Could you check a few things on this model? Use its own coordinates, in mm. A direction names the side the tool comes from. Round coordinates to 2 decimals unless told otherwise and drop trailing zeros. Loops run counter-clockwise (first coordinate to the right, second up) from the corner with the lowest first, then second, coordinate; pieces in that order, holes last. Notation, with made-up numbers: M 36.25,-33.75 L 73.25,-33.75 A24 cw 73.25,2.25 Z; hole C -27,-8.75 d10. An arc over 180 degrees is marked long. Return JSON: item names as keys, results as strings. Group by question number.
```python
from build123d import *

# Parameters (mm, degrees)
F1_DEPTH = 6.35
F2_R     = 2.38125
F3_DEPTH = 6.35


with BuildPart() as f1:
    # F0 (on Top) → F1 (new body)
    with BuildSketch(Plane.XY):
        with BuildLine():
            Line((-9.525, 10.649274), (-6.35, 7.099516))
            ThreePointArc((-6.35, 7.099516), (9.525, 0), (-6.35, -7.099516))
            Line((-6.35, -7.099516), (-9.525, -10.649274))
            ThreePointArc((-9.525, -10.649274), (14.2875, 0), (-9.525, 10.649274))
        make_face()
    extrude(amount=F1_DEPTH)

    # F2 (on Top) → F3 (join, through all)
    with BuildSketch(Plane.XY):
        with BuildLine():
            Line((39.330256, 3.175), (13.930256, 3.175))
            ThreePointArc((13.930256, 3.175), (14.2875, 0), (13.930256, -3.175))
            Line((13.930256, -3.175), (39.330256, -3.175))
            ThreePointArc((39.330256, -3.175), (42.505256, 0), (39.330256, 3.175))
        make_face()
        with Locations((20.280256, 0)):
            Circle(F2_R, mode=Mode.SUBTRACT)
        with Locations((26.630256, 0)):
            Circle(F2_R, mode=Mode.SUBTRACT)
        with Locations((32.980256, 0)):
            Circle(F2_R, mode=Mode.SUBTRACT)
        with Locations((39.330256, 0)):
            Circle(F2_R, mode=Mode.SUBTRACT)
    extrude(amount=F3_DEPTH)


solid = f1.part
```
1. I need wall thicknesses on probe 1 along X at (y, z) = (2, 4.75); probe 2 along X at (y, z) = (-0.25, 2.5); probe 3 along Y at (x, z) = (0, 1.5) (1 decimal). Which ranges of each line are inside material? Lowest first, please.
2. If we section it at B-B, the plane y = 0: Give the number of separate pieces and of enclosed holes in the cut face, then the cut area to 3 significant figures.
3. I'm going to push flat-ended pins straight in: pin 1 Ø1.5 at (y, z) = (1, 4) entering from +X; pin 2 Ø2 at (x, z) = (7.5, 3.5) entering from +Y; pin 3 Ø3 at (x, z) = (28, 4.5) entering from -Y (3 decimals). Where does each tip first touch, or does it pass through?
4. On a 3-axis mill with a long thin cutter (end or side, diameter ignored), from which of +Z, -Z, +X, -X, +Y, -Y can I reach the whole of each face in a straight line? I mean faces 4 (the face through (4.535, 13.549, 3.131)), 5 (the face through (-7.915, -8.85, 3.131)). Say none if no direction works.
5. We'd pull the mould along Y, two halves only. Please class faces 1 (the face through (26, -3.175, 3)), 2 (the face through (9.52, 0.31, 3.13)), 3 (the face through (27, 3.175, 3)): +Y half, -Y half, draft (parallel to the pull), parting line (faces both ways), or undercut.
6. If we section it at D-D, the plane y = -8: Please give me the cut outline in (x, z), then the cut area to 3 significant figures.
Geometry results:
{
 "1": {"probe 1": "9.31 to 18.99, 21.57 to 25.34, 27.92 to 31.69, 34.27 to 38.04, 40.62 to 41.8", "probe 2": "9.52 to 17.91, 22.65 to 24.26, 29 to 30.61, 35.35 to 36.96, 41.7 to 42.5", "probe 3": "-14.3 to -9.5, 9.5 to 14.3"},
 "2": {"separate pieces": "5", "enclosed holes": "0", "area": "88.5 mm^2"},
 "3": {"pin 1": "x = 42.5", "pin 2": "y = 12.72", "pin 3": "y = -3.175"},
 "4": {"face 4": "+Z, -Z, +Y", "face 5": "+Z, -Z, -X"},
 "5": {"face 1": "-Y half", "face 2": "undercut", "face 3": "+Y half"},
 "6": {"outline": "M -7.16,0 L -5.17,0 L -5.17,6.35 L -7.16,6.35 Z; M 5.17,0 L 11.84,0 L 11.84,6.35 L 5.17,6.35 Z", "area": "55.0 mm^2"}
}
